Verification items for this drawing (mm, ordinates from the low corner). Round coordinates to 2 decimals unless told otherwise and drop trailing zeros. Order: outer loops, then holes, each group sorted by start corner. A loop starts at its lowest first (then second) coordinate and runs counter-clockwise, first axis right, second up. Notation, with made-up numbers: M -20,38.5 L -10,38.5 A34 cw -10,77.5 Z; hole C 6.25,-38 d2. An arc over 180 degrees is marked long. Use CSV: the item, a comma, the result in double quotes. Start each with the question number.
Q1. Sectioned sample at A-A (y = 3.55). State how many separate pieces and enclosed holes the cut face has, and give its area (3 significant figures).
Q2. Scan lines: line 1 (Z direction, x = 45, y = 2.6); line 2 (Z direction, x = 180, y = 1.6); line 3 (X direction, y = 1.8, z = 82). Record each from-to range of solid material in increasing order.
Q3. Sectioned sample at B-B (x = 113). Enter the section's corners in (y, z).
Q4. Gauge pin test, flat end, axial feed: pin 1 Ø1.5 at (x, y) = (116.5, 1.5) entering from -Z. Record the tip position at first contact, or that the pin passes through.
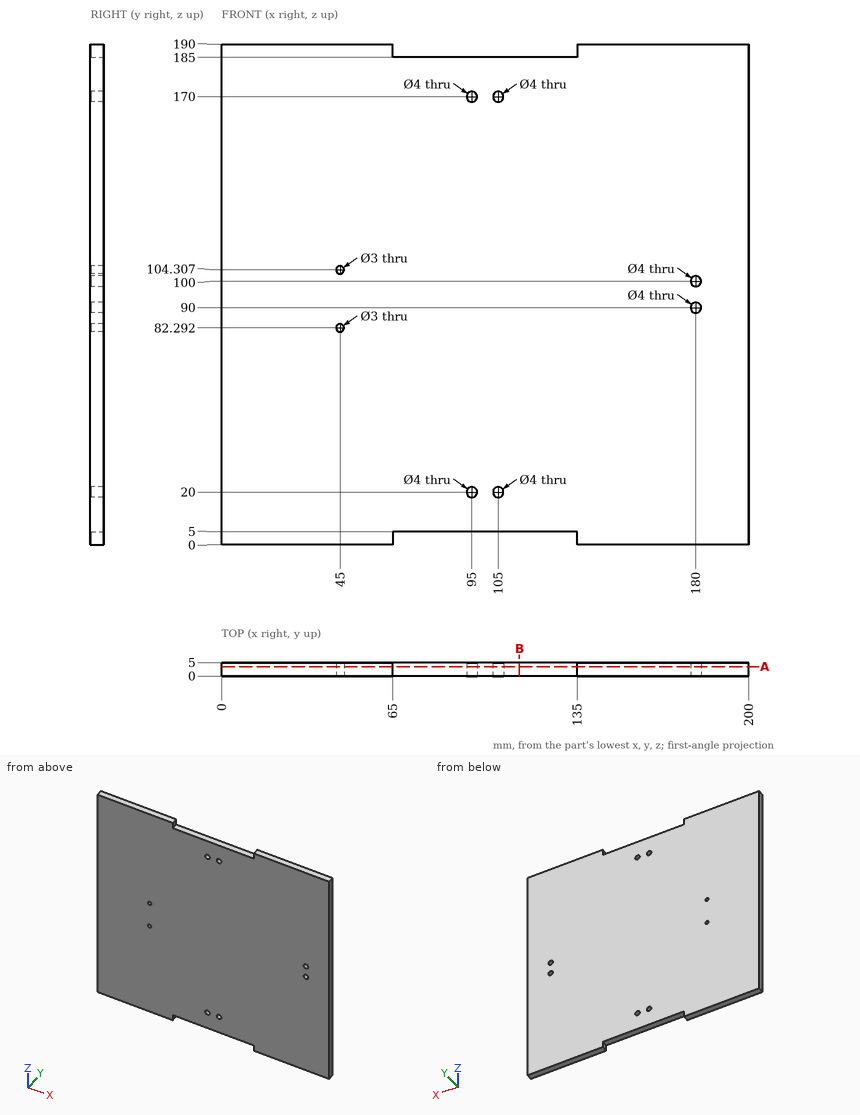
Verdict:
1,separate pieces,"1"
1,enclosed holes,"8"
1,area,"37,200 mm²"
2,line 1,"z = 0 to 80.79, 83.79 to 102.81, 105.81 to 190"
2,line 2,"z = 0 to 88, 92 to 98, 102 to 190"
2,line 3,"x = 0 to 43.53, 46.47 to 200"
3,outline,"M 0,5 L 5,5 L 5,185 L 0,185 Z"
4,pin 1,"stops at z = 5"
